Work out the finished part from the listing and answer in its coordinate system (mm). Round coordinates to 2 decimals unless told otherwise and drop trailing zeros. Order: outer loops, then holes, each group sorted by start corner. A loop starts at its lowest first (then second) coordinate and runs counter-clockwise, first axis right, second up. Notation, with made-up numbers: M -26,-27 L 14,-27 A20 ccw 14,-16 Z; hole C 62.5,41 d10. An arc over 180 degrees is marked long. Return JSON: item names as keys, results as strings.
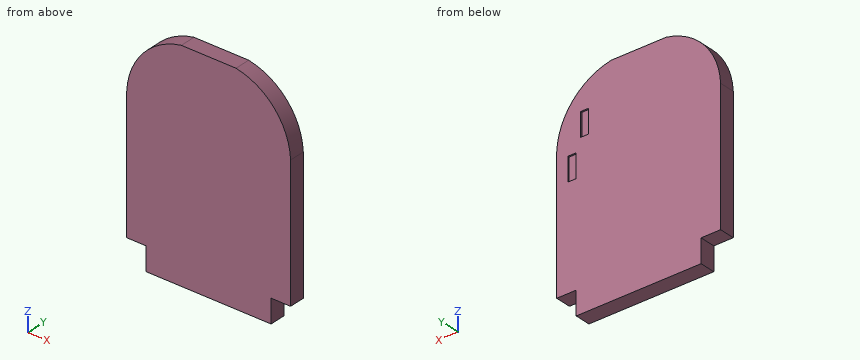
from build123d import *

# Parameters (mm, degrees)
EXTRUDE_1_DEPTH     = 2
SKETCH_2_W          = 1
SKETCH_2_H          = 3
CUT_EXTRUDE_1_DEPTH = 0.2


with BuildPart() as part:
    # 草图1 → 凸台-拉伸1 (new body)
    with BuildSketch(Plane(origin=(0, 0, 0), x_dir=(1, 0, 0), z_dir=(0, 1, 0))):
        with BuildLine():
            Line((-8, 14), (8, 14))
            Line((8, 14), (8, 11))
            Line((8, 11), (10.5, 11))
            Line((10.5, 11), (10.5, -6))
            ThreePointArc((10.5, -6), (8.403124237, -11.227733708), (3.5, -14))
            Line((3.5, -14), (-3.5, -14))
            ThreePointArc((-3.5, -14), (-8.403124237, -11.227733708), (-10.5, -6))
            Line((-10.5, -6), (-10.5, 11))
            Line((-10.5, 11), (-8, 11))
            Line((-8, 11), (-8, 14))
        make_face()
    extrude(amount=EXTRUDE_1_DEPTH)

    # 草图2 → 切除-拉伸1 (cut)
    with BuildSketch(Plane(origin=(0, 2, 0), x_dir=(1, 0, 0), z_dir=(0, 1, 0))):
        with Locations((8.561436861, -3.449742869)):
            Rectangle(SKETCH_2_W, SKETCH_2_H)
        with Locations((6.933076326, -8.027614823)):
            Rectangle(SKETCH_2_W, SKETCH_2_H)
    extrude(amount=-CUT_EXTRUDE_1_DEPTH, mode=Mode.SUBTRACT)


solid = part.part
Item 1: Consider line 1 along X through (y, z) = (0.2, -12); line 2 along Z through (x, y) = (-9.5, 1.95); line 3 along Z through (x, y) = (5, 1.15). Determine where each line is inside the solid, lowest interval first. Write a range as [from, to].
Output:
{"line 1": "x = [-8, 8]", "line 2": "z = [-11, 9.64]", "line 3": "z = [-14, 13.59]"}
Item 2: Find section A-A (y = 0.6). Determine the outline of the cut face in (x, z) (3 decimals), plus the area to 3 significant figures.
Output:
{"outline": "M -10.5,-11 L -8,-11 L -8,-14 L 8,-14 L 8,-11 L 10.5,-11 L 10.5,6 A8.508 ccw 3.5,14 L -3.5,14 A8.508 ccw -10.5,6 Z", "area": "544 mm^2"}
Item 3: Each of these flat-tipped pins is pushed along its axis until it touches: pin 1 (1 mm diameter, centred on y = 1, z = -13, fed in from +X); pin 2 (0.8 mm diameter, centred on x = 7, z = 8.5, fed in from +Y). Where does it stop, or does it pass through?
Output:
{"pin 1": "stops at x = 8", "pin 2": "stops at y = 1.8"}
Item 4: Find section B-B (z = 9). Determine the outline of the cut face in (x, y).
Output:
{"outline": "M -9.81,0 L 9.81,0 L 9.81,2 L 7.43,2 L 7.43,1.8 L 6.43,1.8 L 6.43,2 L -9.81,2 Z"}
Item 5: Find section C-C (x = 5.25). Determine the outline of the cut face in (y, z).
Output:
{"outline": "M 0,-14 L 2,-14 L 2,13.49 L 0,13.49 Z"}
